Job drawing, mm, ordinate dimensions from the low corner. One solid piece. A direction names the side the tool comes from. Coordinates: 2 decimals unless noted, no trailing zeros. Order: outer loops, then holes, each group sorted by start corner. A loop starts at its lowest first (then second) coordinate and runs counter-clockwise, first axis right, second up. Notation, with made-up numbers: (49.5, 82.5) - (66.5, 82.5) arc R18 ccw to (66.5, 113.5) - close; hole circle Ø8 at (12.5, 61.5). An arc over 180 degrees is marked (long way). Use a Markdown table: item, result. Add a question column.
1) Saw through at B-B on x = 7.5. List the corners of the cut face in (y, z), then the cut area to 3 significant figures.
2) Drop flat-ended pins along their axis: P1, Ø3, axis at x = 9, z = 13, coming from the +Y side; P2, Ø5, axis at y = 31.5, z = 11, coming from the +X side; P3, Ø4, axis at x = 10.5, z = 4.5, coming from the +Y side. Give the stop position or say it passes through.
3) Wall check: L1, parallel to Y at x = 11.5, z = 4.25; L2, parallel to Z at x = 9.5, y = 25; L3, parallel to X at y = 9, z = 10.25. Give the ranges that are in metal, low to high. Write a range as [from, to].
4) Saw through at C-C on y = 6. List the corners of the cut face in (x, z), then the cut area to 3 significant figures.
5) Tool access for the marked faces 1 and 2: list every direction of +Z, -Z, +X, -X, +Y, -Y with a clear straight run to the whole face (end or side of a thin tool).
6) Saw through at A-A on z = 7.5. List the corners of the cut face in (x, y), then the cut area to 3 significant figures.
7) Saw through at D-D on y = 19.5. List the corners of the cut face in (x, z), then the cut area to 3 significant figures.
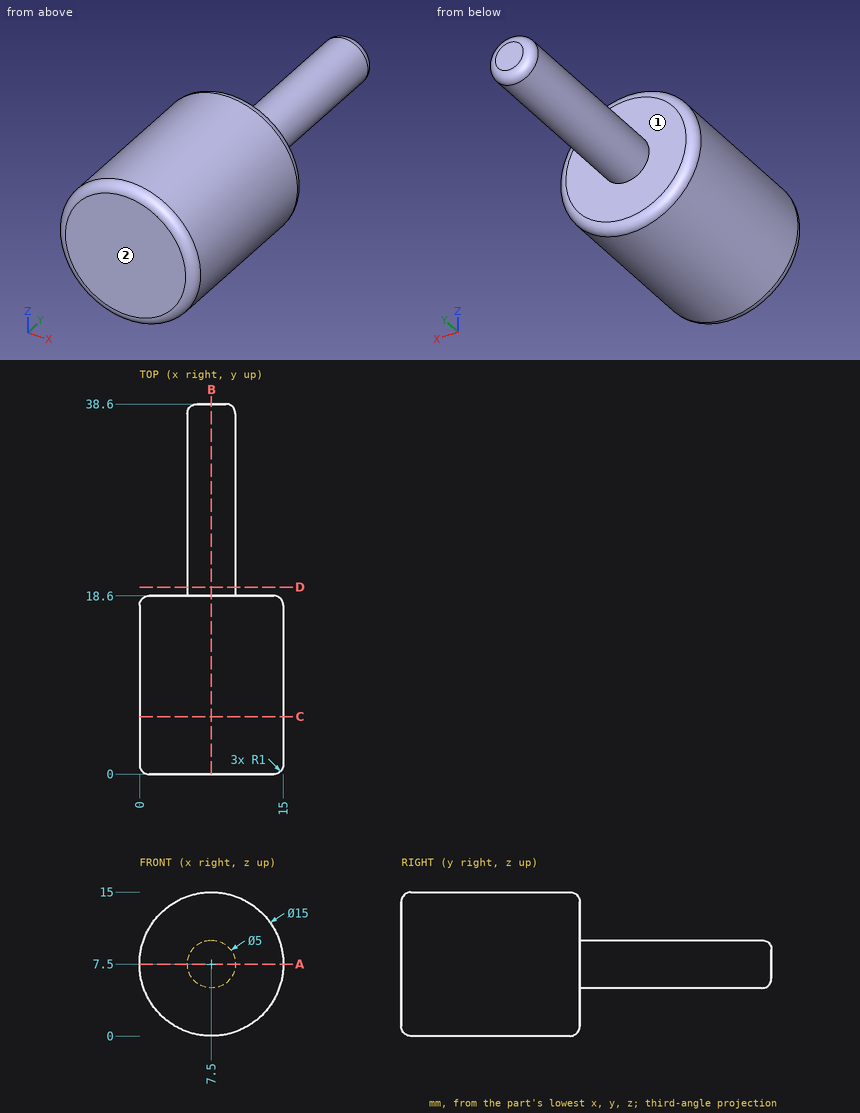
Results are:
| question | item | result |
|---|---|---|
| 1 | outline | (0, 1) arc R1 ccw to (1, 0) - (17.6, 0) arc R1 ccw to (18.6, 1) - (18.6, 5) - (37.6, 5) arc R1 ccw to (38.6, 6) - (38.6, 9) arc R1 ccw to (37.6, 10) - (18.6, 10) - (18.6, 14) arc R1 ccw to (17.6, 15) - (1, 15) arc R1 ccw to (0, 14) - close |
| 1 | area | 378 mm2 |
| 2 | P1 | y = 18.6 |
| 2 | P2 | x = 9.79 |
| 2 | P3 | y = 38.27 |
| 3 | L1 | [0, 18.6] |
| 3 | L2 | [6, 9] |
| 3 | L3 | [0.52, 14.48] |
| 4 | outline | circle Ø15 at (7.5, 7.5) |
| 4 | area | 177 mm2 |
| 5 | face 1 | +Y |
| 5 | face 2 | +Z, -Z, +X, -X, -Y |
| 6 | outline | (0, 1) arc R1 ccw to (1, 0) - (14, 0) arc R1 ccw to (15, 1) - (15, 17.6) arc R1 ccw to (14, 18.6) - (10, 18.6) - (10, 37.6) arc R1 ccw to (9, 38.6) - (6, 38.6) arc R1 ccw to (5, 37.6) - (5, 18.6) - (1, 18.6) arc R1 ccw to (0, 17.6) - close |
| 6 | area | 378 mm2 |
| 7 | outline | circle Ø5 at (7.5, 7.5) |
| 7 | area | 19.6 mm2 |
